Drawing for the job (mm, zero at the part's lowest x, y, z). A direction names the side the tool comes from. Round coordinates to 2 decimals unless told otherwise and drop trailing zeros. Loops run counter-clockwise (first coordinate to the right, second up) from the corner with the lowest first, then second, coordinate; pieces in that order, holes last. Notation, with made-up numbers: (-6.75, -26.5) -> (30.25, -26.5) arc R19 ccw to (30.25, -20.5) -> close; hole circle Ø5 at (5.25, 35.25). An arc over 180 degrees is marked (long way). Put each result on its own line as item: value. Start each with the question number.
Item 1: Tool access for the marked faces 1, 2 and 3: list every direction of +Z, -Z, +X, -X, +Y, -Y with a clear straight run to the whole face (end or side of a thin tool).
Item 2: Cut at D-D, the plane x = 18.5. List the corners of the cut face in (y, z), plus the area to 3 significant figures.
Item 3: Drill centre lines: probe 1 along Y at (x, z) = (6.25, 7); probe 2 along Z at (x, y) = (11.5, 7). Where is each one in solid material? Low to high. Write a range as [from, to].
Item 4: Flat gauge pins, fed straight in: pin 1 Ø1.5 at (y, z) = (6.5, 7.5) entering from -X; pin 2 Ø3 at (y, z) = (8, 11) entering from +X; pin 3 Ø4 at (x, y) = (21.5, 10) entering from -Z. Where does each tip first touch, or does it go through?
Item 5: Cut at C-C, the plane x = 7. List the corners of the cut face in (y, z).
Item 6: Cut at A-A, the plane z = 7. List the corners of the cut face in (x, y), plus the area to 4 significant figures.
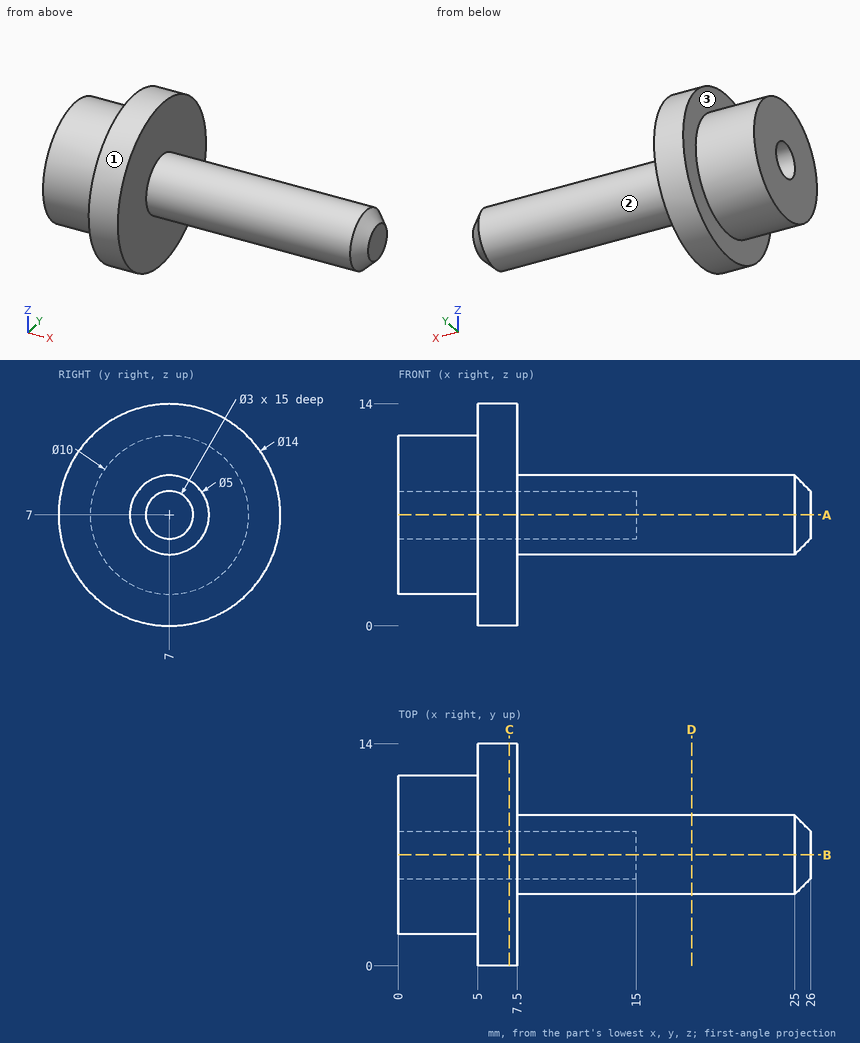
Reply:
1. face 1: +X, -X
1. face 2: +X
1. face 3: -X
2. outline: circle Ø5 at (7, 7)
2. area: 19.6 mm^2
3. probe 1: y = [0, 5.5], [8.5, 14]
3. probe 2: z = [4.5, 5.5], [8.5, 9.5]
4. pin 1: stops at x = 15
4. pin 2: stops at x = 7.5
4. pin 3: stops at z = 4.71
5. outline: circle Ø14 at (7, 7); hole circle Ø3 at (7, 7)
6. outline: (0, 2) -> (5, 2) -> (5, 0) -> (7.5, 0) -> (7.5, 4.5) -> (25, 4.5) -> (26, 5.5) -> (26, 8.5) -> (25, 9.5) -> (7.5, 9.5) -> (7.5, 14) -> (5, 14) -> (5, 12) -> (0, 12) -> (0, 8.5) -> (15, 8.5) -> (15, 5.5) -> (0, 5.5) -> close
6. area: 131.5 mm^2
